The listing builds one solid part. Answer for the finished solid, in the listing's coordinates (mm). A direction names the side the tool comes from. Coordinates: 2 decimals unless noted, no trailing zeros. Loops run counter-clockwise (first coordinate to the right, second up) from the corner with the lowest first, then second, coordinate; pieces in that order, holes last. Notation, with made-up numbers: M 55,16 L 60,16 A13 ccw 60,24 Z; hole C 27.5,-14.75 d8. An arc over 180 degrees is marked long. Answer as a JSON object with one key per item and string values. Group by question number.
1. Given pin 1 (6 mm diameter, centred on x = 26.5, z = 32.5, fed in from +Y); pin 2 (2.5 mm diameter, centred on x = 2.5, y = -8, fed in from +Z); pin 3 (1.5 mm diameter, centred on y = -11.5, z = -3, fed in from +X), each flat-ended and moving along its own axis, determine where each tip first touches the part or whether it passes through.
2. A cutting plane is placed at D-D on y = -4. Give the vertices of the cut face in (x, z).
3. Straight lines are drawn through the part: L1, parallel to X at y = -25, z = 51; L2, parallel to Z at x = 11, y = -24; L3, parallel to Z at x = 25.5, y = -12.5. For each, find the intervals that lie inside material, in ascending order.
4. A cutting plane is placed at A-A on z = 22.5. Give the vertices of the cut face in (x, y) (3 decimals).
5. A cutting plane is placed at B-B on y = -24. Give the vertices of the cut face in (x, z).
6. Determine the mould class of faces 3 (the face through (-53.406, -41, -1)), 4 (the face through (-19, -16, 24.437)), 5 (the face through (3, -8, 55.771)) for opening direction Z: released by +Z, released by -Z, zero draft, split by the parting line, or undercut.
7. For faces 1 (the face through (3, 0, 0)), 2 (the face through (38.428, -24, -1)), determine the directions among +Z, -Z, +X, -X, +Y, -Y from which every point of the face is accessible in a straight line to the end or side of a thin tool.
8. A cutting plane is placed at C-C on x = 17. Give the vertices of the cut face in (y, z) (3 decimals), and give its area (3 significant figures).
from build123d import *

# Parameters (mm, degrees)
F0_W     = 76.8568962812
F0_H     = 111.5410327911
F1_DEPTH = 25.4
F2_W     = 38.4284481406
F2_H     = 31.9251716137
F2_H_2   = 42.9610349238
F2_H_3   = 36.6548262537
F3_DEPTH = 9.525
F4_W     = 106.8113818765
F4_H     = 128.8831084967
F5_DEPTH = 50.8
F6_DEPTH = 31.75
F7_W     = 5.1237931475
F7_H     = 31.333964318
F7_H_2   = 4.72965464
F7_H_3   = 40.0050021708
F7_W_2   = 32.7134476975
F7_H_4   = 4.3355170637
F7_W_3   = 38.0343087018
F7_W_4   = 32.5163798407
F8_DEPTH = 50.8


with BuildPart() as f1:
    # F0 (on Front) → F1 (new body)
    with BuildSketch(Plane.XZ):
        Rectangle(F0_W, F0_H)
    extrude(amount=F1_DEPTH)

    # F2 (on face) → F3 (cut)
    with BuildSketch(Plane.XZ.offset(25.4)):
        with Locations((-19.2142240703, 39.8079305887)):
            Rectangle(F2_W, F2_H)
        with Locations((19.2142240703, 39.8079305887)):
            Rectangle(F2_W, F2_H)
        with Locations((19.2142240703, 2.36482732)):
            Rectangle(F2_W, F2_H_2)
        with Locations((-19.2142240703, 2.36482732)):
            Rectangle(F2_W, F2_H_2)
        with Locations((-19.2142240703, -37.4431032687)):
            Rectangle(F2_W, F2_H_3)
        with Locations((19.2142240703, -37.4431032687)):
            Rectangle(F2_W, F2_H_3)
    extrude(amount=-F3_DEPTH, mode=Mode.SUBTRACT)

    # F4 (on face) → F5 (join)
    with BuildSketch(Plane.XZ.offset(15.875)):
        Rectangle(F4_W, F4_H)
    extrude(amount=F5_DEPTH)

    # F6 (cut): a face of the model
    f6_faces = [f1.faces().sort_by_distance(p)[0] for p in [
        (0, 0, 0),
    ]]
    extrude(f6_faces, amount=-F6_DEPTH, mode=Mode.SUBTRACT)

    # F7 (on Front) → F8 (join)
    with BuildSketch(Plane.XZ):
        with Locations((2.5618965738, 40.1035342366)):
            Rectangle(F7_W, F7_H)
        with Locations((2.5618965738, 22.0717247576)):
            Rectangle(F7_W, F7_H_2)
        Polygon((0, 19.7068974376), (0, 24.4365520775), (-37.4431051314, 24.4365520775), (-38.0343087018, 24.4365520775), (-38.0343087018, 19.7068974376), align=None)
        with Locations((2.5618965738, -0.2956036478)):
            Rectangle(F7_W, F7_H_3)
        with Locations((21.4805169962, 22.0717247576)):
            Rectangle(F7_W_2, F7_H_2)
        with Locations((2.5618965738, -22.4658632651)):
            Rectangle(F7_W, F7_H_4)
        with Locations((-19.0171543509, -22.4658632651)):
            Rectangle(F7_W_3, F7_H_4)
        Polygon((5.1237931475, -24.633621797), (0, -24.633621797), (0, -54.5881018043), (0, -55.9675879776), (5.1237931475, -55.9675879776), align=None)
        with Locations((21.3819830678, -22.4658632651)):
            Rectangle(F7_W_4, F7_H_4)
    extrude(amount=F8_DEPTH)


solid = f1.part
From the geometry:
{
 "1": {"pin 1": "stops at y = -31.75", "pin 2": "stops at z = 55.77", "pin 3": "stops at x = 5.12"},
 "2": {"outline": "M -38.03,-24.63 L 0,-24.63 L 0,-55.97 L 5.12,-55.97 L 5.12,-24.63 L 37.64,-24.63 L 37.64,-20.3 L 5.12,-20.3 L 5.12,19.71 L 37.84,19.71 L 37.84,24.44 L 5.12,24.44 L 5.12,55.77 L 0,55.77 L 0,24.44 L -38.03,24.44 L -38.03,19.71 L 0,19.71 L 0,-20.3 L -38.03,-20.3 Z"},
 "3": {"L1": "x = -53.41 to -38.43, 0 to 5.12, 38.43 to 53.41", "L2": "z = -64.44 to -55.77, -24.63 to -20.3, 19.71 to 24.44, 55.77 to 64.44", "L3": "z = -24.63 to -20.3, 19.71 to 24.44"},
 "4": {"outline": "M -53.406,-66.675 L 53.406,-66.675 L 53.406,-15.875 L 38.428,-15.875 L 38.428,-31.75 L 37.837,-31.75 L 37.837,0 L -38.034,0 L -38.034,-31.75 L -38.428,-31.75 L -38.428,-15.875 L -53.406,-15.875 Z"},
 "5": {"outline": "M -53.41,-64.44 L 53.41,-64.44 L 53.41,64.44 L -53.41,64.44 Z; hole M -38.43,-55.77 L 0,-55.77 L 0,-24.63 L -38.03,-24.63 L -38.03,-20.3 L 0,-20.3 L 0,19.71 L -38.03,19.71 L -38.03,24.44 L 0,24.44 L 0,55.77 L -38.43,55.77 Z; hole M 5.12,-55.77 L 38.43,-55.77 L 38.43,55.77 L 5.12,55.77 L 5.12,24.44 L 37.84,24.44 L 37.84,19.71 L 5.12,19.71 L 5.12,-20.3 L 37.64,-20.3 L 37.64,-24.63 L 5.12,-24.63 Z"},
 "6": {"face 3": "zero draft", "face 4": "undercut", "face 5": "released by +Z"},
 "7": {"face 1": "+Z, -Z, +X, -X, +Y", "face 2": "+Y"},
 "8": {"outline": "M -66.675,-64.442 L -15.875,-64.442 L -15.875,-55.771 L -31.75,-55.771 L -31.75,-24.634 L 0,-24.634 L 0,-20.298 L -31.75,-20.298 L -31.75,19.707 L 0,19.707 L 0,24.437 L -31.75,24.437 L -31.75,55.771 L -15.875,55.771 L -15.875,64.442 L -66.675,64.442 Z", "area": "5,060 mm²"}
}
